```python
from build123d import *

# Parameters (mm, degrees)
BOSS_EXTRUDE2_DEPTH       = 152.4
F_4_CLEARANCE_HOLE1_D     = 3.2639
F_4_CLEARANCE_HOLE1_DEPTH = 1.524
F_4_CLEARANCE_HOLE1_TIP   = 0.980574487


with BuildPart() as part:
    # Sketch2 → Boss-Extrude2 (new body)
    with BuildSketch(Plane.XY):
        with BuildLine():
            Line((-0.508, -4.915254952), (-0.508, 6.746875))
            Line((-0.508, 6.746875), (0.508, 6.746875))
            Line((0.508, 6.746875), (0.508, -6.746875))
            ThreePointArc((0.508, -6.746875), (-3.538990731, -7.794143829), (-0.508, -4.915254952))
        make_face()
    extrude(amount=BOSS_EXTRUDE2_DEPTH)

    # #4 Clearance Hole1
    with Locations(Plane.ZY.offset(0.508)):
        with Locations((25.4, 0), (76.2, 0), (127, 0)):
            Hole(F_4_CLEARANCE_HOLE1_D / 2, depth=F_4_CLEARANCE_HOLE1_DEPTH)
            with Locations((0, 0, -(F_4_CLEARANCE_HOLE1_DEPTH + F_4_CLEARANCE_HOLE1_TIP / 2))):  # 118° drill point
                Cone(0, F_4_CLEARANCE_HOLE1_D / 2, F_4_CLEARANCE_HOLE1_TIP, mode=Mode.SUBTRACT)


solid = part.part
```
The listing builds one solid part. Answer for the finished solid, in the listing's coordinates (mm). Round coordinates to 2 decimals unless told otherwise and drop trailing zeros. Loops run counter-clockwise (first coordinate to the right, second up) from the corner with the lowest first, then second, coordinate; pieces in that order, holes last.
Q1. Section A-A, the plane y = 0 is taken. Determine the outline of the cut face in (x, z), then the cut area to 3 significant figures.
Q2. Find the intervals of material crossed by line 1 (X direction, y = 2, z = 55); line 2 (Z direction, x = -0.2, y = -0.5); line 3 (Y direction, x = 0.2, z = 127), in increasing order.
Q3. Section D-D, the plane x = -2.2 is taken. Determine the outline of the cut face in (y, z).
Q4. Given pin 1 Ø4 at (y, z) = (0, 76.2) entering from +X; pin 2 Ø1 at (y, z) = (2.5, 83.5) entering from -X; pin 3 Ø3 at (y, z) = (0, 25.4) entering from +X, each flat-ended and moving along its own axis, determine where each tip first touches the part or whether it passes through.
Q5. Section C-C, the plane z = 89.5 is taken. Determine the outline of the cut face in (x, y), then the cut area to 3 significant figures.
Q6. For a pull along Z with two mould halves and no side action, classify faces 1 (the face through (0.508, 2, 75)), 2 (the face through (0, -3, 0)), 3 (the face through (0.007, -0.625, 74.692)), 4 (the face through (0.007, -0.625, 125.492)) as released by +Z, released by -Z, zero draft, split by the parting line, or undercut.
Q7. Section B-B, the plane z = 25.4 is taken. Determine the outline of the cut face in (x, y).
Completed:
1. outline: (-0.51, 0) - (0.51, 0) - (0.51, 23.77) - (-0.51, 23.77) - close; (-0.51, 27.03) - (0.51, 27.03) - (0.51, 74.57) - (-0.51, 74.57) - close; (-0.51, 77.83) - (0.51, 77.83) - (0.51, 125.37) - (-0.51, 125.37) - close; (-0.51, 128.63) - (0.51, 128.63) - (0.51, 152.4) - (-0.51, 152.4) - close
1. area: 145 mm2
2. line 1: x = -0.51 to 0.51
2. line 2: z = 0 to 23.85, 26.95 to 74.65, 77.75 to 125.45, 128.55 to 152.4
2. line 3: y = -7.86 to -1.63, 1.63 to 6.75
3. outline: (-8.83, 0) - (-4.66, 0) - (-4.66, 152.4) - (-8.83, 152.4) - close
4. pin 1: stops at x = 0.51
4. pin 2: stops at x = -0.51
4. pin 3: passes through
5. outline: (-0.51, -4.92) arc R2.16 ccw (long way) to (0.51, -6.75) - (0.51, 6.75) - (-0.51, 6.75) - close
5. area: 27.0 mm2
6. face 1: zero draft
6. face 2: released by -Z
6. face 3: undercut
6. face 4: undercut
7. outline: (-0.51, -4.92) arc R2.16 ccw (long way) to (0.51, -6.75) - (0.51, -1.63) - (-0.51, -1.63) - close; (-0.51, 1.63) - (0.51, 1.63) - (0.51, 6.75) - (-0.51, 6.75) - close
